Verification items for the finished model (mm, model axes). A direction names the side the tool comes from. Give positions to 0.01 mm unless a question says otherwise; leave off trailing zeros. Write each loop counter-clockwise with the first axis right and the second up, starting at its lowest first coordinate (ties: lowest second). Pieces come first, ordered by that corner, then holes. Notation, with made-up numbers: (38.25, 55) -> (94.25, 55) arc R18 ccw to (94.25, 68) -> close; hole circle Ø5 at (1.25, 80.5). An arc over 180 degrees is marked (long way). Use one line per item in the form item = value. Start each with the question number.
(1) Scan lines: L1, parallel to Z at x = 0.35, y = -2.5; L2, parallel to Y at x = 0.5, z = 1; L3, parallel to Y at x = 0.7, z = 5.5. Record each from-to range of solid material in increasing order.
(2) Release check for a two-part mould opening along Y. For faces 5 (the face through (1.5, -10.5, 0)), 6 (the face through (1, 17.5, 0)), 7 (the face through (1, -14, 8)) record: pulls with the +Y half, pulls with the -Y half, needs draft (parallel to the pull), parting line crosses it, or undercut.
(3) Depth check by flat-ended pin: pin 1 Ø0.9 at (x, z) = (2, 7.5) entering from +Y; pin 2 Ø1 at (x, y) = (0.5, 6) entering from +Z; pin 3 Ø0.9 at (x, y) = (1, 2) entering from -Z; pin 4 Ø1 at (y, z) = (7.5, 5) entering from -X. Enter the tip coordinate at first touch or a pass-through.
(4) Section check B-B, the plane z = 0. Record the cut outline in (x, y).
(5) Set-up check for faces 1 (the face through (2, -12.5, 7)), 2 (the face through (1.5, 15.5, 0)), 3 (the face through (1.52, -16.9, 7.43)), 4 (the face through (2, -12.5, -7)): record each of +Z, -Z, +X, -X, +Y, -Y from which the full face is reachable in a straight line by a thin tool's end or side.
(6) Section check C-C, the plane x = 1.6. Record the cut outline in (y, z).
(7) Section check A-A, the plane y = 7. Record the cut outline in (x, z), plus the area to 3 significant figures.
Autodesk Inventor part; units mm, degrees
ref_plane "YZ Plane" through (0, 0, 0) normal (1, 0, 0) x (0, 1, 0)
ref_plane "XZ Plane" through (0, 0, 0) normal (0, 1, 0) x (-1, 0, 0)
ref_plane "XY Plane" through (0, 0, 0) normal (0, 0, 1) x (1, 0, 0)
sketch "Sketch1" plane through (0, 0, 0) normal (1, 0, 0) x (0, 1, 0)
  line L0 (17.5, 8) -> (-17.5, 8)
  line L1 (-17.5, 8) -> (-17.5, -8)
  line L2 (-17.5, -8) -> (17.5, -8)
  line L3 (17.5, -8) -> (17.5, 8)
  line L4 (17.5, 8) -> (-17.5, -8) construction
  line L5 (-17.5, 8) -> (17.5, -8) construction
  point P0 (0, 0)
  dimension "d0" = 35
  dimension "d1" = 16
extrude "Extrusion1" add sketch "Sketch1" along normal blind 3
sketch "Sketch2" plane through (3, 0, 0) normal (1, 0, 0) x (0, 0, -1)
  line L0 (-8, 17.5) -> (-8, -17.5) construction
  line L1 (-8, -12.5) -> (7.9898, -12.5) construction
  line L2 (-8, -17.5) -> (8, -17.5) construction
  line L3 (8, 17.5) -> (-8, 17.5) construction
  line L4 (-8, 17.5) -> (7.9898, -12.5) construction
  line L5 (8, -17.5) -> (8, 17.5) construction
  line L6 (8, 17.5) -> (-8, -12.5) construction
  line L7 (0, 14) -> (0, -9) construction
  line L8 (-1.5, 14) -> (-1.5, -9)
  line L9 (1.5, -9) -> (1.5, 14)
  arc A0 (1.5, 14) -> (-1.5, 14) centre (0, 14) ccw
  arc A1 (-1.5, -9) -> (1.5, -9) centre (0, -9) ccw
  line L10 (6.25, -12.5) -> (8, -12.5)
  line L11 (8, -12.5) -> (8, 17.5)
  line L12 (8, 17.5) -> (6.25, 17.5)
  line L13 (6.25, 17.5) -> (6.25, -12.5)
  line L14 (-6.25, -12.5) -> (-8, -12.5)
  line L15 (-8, -12.5) -> (-8, 17.5)
  line L16 (-8, 17.5) -> (-6.25, 17.5)
  line L17 (-6.25, 17.5) -> (-6.25, -12.5)
  point P0 (0, 0)
  point P1 (0, 2.5)
  point P2 (-7.9898, -12.5)
  dimension "d4" = 5
  dimension "d5" = 3
  dimension "d6" = 23
  dimension "d9" = 6.25
extrude "Extrusion2" cut sketch "Sketch2" against normal through all
fillet "Fillet1" radius 2 4 edges at (1.5, 17.5, 6.25) (1.5, 17.5, -6.25) (1.5, -17.5, 8) (1.5, -17.5, -8)
properties part number "Ga mica 5mm"
Completed:
q1.L1 = -6.25 to -1.5, 1.5 to 6.25
q1.L2 = -17.5 to -10.12, 15.12 to 17.5
q1.L3 = -17.5 to 17.06
q2.face_5 = undercut
q2.face_6 = pulls with the +Y half
q2.face_7 = needs draft
q3.pin_1 = -12.5
q3.pin_2 = 6.25
q3.pin_3 = -6.25
q3.pin_4 = 0
q4.outline = (0, -17.5) -> (3, -17.5) -> (3, -10.5) -> (0, -10.5) -> close; (0, 15.5) -> (3, 15.5) -> (3, 17.5) -> (0, 17.5) -> close
q5.face_1 = +Z, +X, -X, +Y
q5.face_2 = +X, -X
q5.face_3 = +Z, +X, -X, -Y
q5.face_4 = -Z, +X, -X, +Y
q6.outline = (-17.5, -6) arc R2 ccw to (-15.5, -8) -> (-12.5, -8) -> (-12.5, -6.25) -> (15.5, -6.25) arc R2 ccw to (17.5, -4.25) -> (17.5, 4.25) arc R2 ccw to (15.5, 6.25) -> (-12.5, 6.25) -> (-12.5, 8) -> (-15.5, 8) arc R2 ccw to (-17.5, 6) -> close; hole (-9, -1.5) -> (14, -1.5) arc R1.5 ccw to (14, 1.5) -> (-9, 1.5) arc R1.5 ccw to start
q7.outline = (0, -6.25) -> (3, -6.25) -> (3, -1.5) -> (0, -1.5) -> close; (0, 1.5) -> (3, 1.5) -> (3, 6.25) -> (0, 6.25) -> close
q7.area = 28.5 mm²
